```python
from build123d import *

# Parameters (mm, degrees)
SKETCH_1_W               = 90
SKETCH_1_H               = 20
EXTRUDE_1_DEPTH          = 5
SKETCH_4_R               = 13
SKETCH_4_R_2             = 3.75
SKETCH_4_R_3             = 1.8
EXTRUDE_3_DEPTH          = 5
SKETCH_3_R               = 1.8
CUT_EXTRUDE_1_DEPTH      = 48.106262853
SKETCH_4_3_R             = 3.75
SKETCH_4_3_R_2           = 1.8
CUT_EXTRUDE_3_DEPTH      = 48.106262853
EXTRUDE_4_DEPTH          = 10
SKETCH_8_W               = 46.403712297
SKETCH_8_H               = 9.925238464
SKETCH_8_H_2             = 7.991750451
CUT_EXTRUDE_4_DEPTH      = 10
CUT_EXTRUDE_5_DEPTH      = 10
CUT_EXTRUDE_5_DEPTH_BACK = 50.183330509
CUT_EXTRUDE_6_DEPTH      = 10
EXTRUDE_5_DEPTH          = 0.5


with BuildPart() as part:
    # ｽｹｯﾁ1 → ﾎﾞｽ - 押し出し1 (new body)
    with BuildSketch(Plane.XY):
        Rectangle(SKETCH_1_W, SKETCH_1_H)
    extrude(amount=EXTRUDE_1_DEPTH)

    # ｽｹｯﾁ4 → ﾎﾞｽ - 押し出し3 (add)
    with BuildSketch(Plane.XY.offset(5)):
        Circle(SKETCH_4_R)
        Circle(SKETCH_4_R_2, mode=Mode.SUBTRACT)
        with Locations((0, 8.2)):
            Circle(SKETCH_4_R_3, mode=Mode.SUBTRACT)
        with Locations((0, -8.195848947)):
            Circle(SKETCH_4_R_3, mode=Mode.SUBTRACT)
    extrude(amount=-EXTRUDE_3_DEPTH)

    # ｽｹｯﾁ3 → ｶｯﾄ - 押し出し1 (cut, through all)
    with BuildSketch(Plane.XY.offset(5)):
        with Locations((-40, 0)):
            Circle(SKETCH_3_R)
        with Locations((-17, 0)):
            Circle(SKETCH_3_R)
        with Locations((17, 0)):
            Circle(SKETCH_3_R)
        with Locations((40, 0)):
            Circle(SKETCH_3_R)
    extrude(amount=-CUT_EXTRUDE_1_DEPTH, mode=Mode.SUBTRACT)

    # ｽｹｯﾁ4<3> → ｶｯﾄ - 押し出し3 (cut, through all)
    with BuildSketch(Plane.XY.offset(5)):
        Circle(SKETCH_4_3_R)
        with Locations((0, 8.2)):
            Circle(SKETCH_4_3_R_2)
        with Locations((0, -8.195848947)):
            Circle(SKETCH_4_3_R_2)
    extrude(amount=-CUT_EXTRUDE_3_DEPTH, mode=Mode.SUBTRACT)

    # ｽｹｯﾁ6 → ﾎﾞｽ - 押し出し4 (add)
    with BuildSketch(Plane(origin=(0, 0, 0), x_dir=(-1, 0, 0), z_dir=(0, 0, -1))):
        with BuildLine():
            Line((-19.539767143, 10), (-9.797958971, 10))
            ThreePointArc((-9.797958971, 10), (-14, 0), (-9.797958971, -10))
            Line((-9.797958971, -10), (-19.539767143, -10))
            ThreePointArc((-19.539767143, -10), (-21.95, 0), (-19.539767143, 10))
        make_face()
        with BuildLine():
            Line((9.797958971, 10), (19.539767143, 10))
            ThreePointArc((19.539767143, 10), (21.95, 0), (19.539767143, -10))
            Line((19.539767143, -10), (9.797958971, -10))
            ThreePointArc((9.797958971, -10), (14, 0), (9.797958971, 10))
        make_face()
    extrude(amount=EXTRUDE_4_DEPTH)

    # ｽｹｯﾁ8 → ｶｯﾄ - 押し出し4 (cut)
    with BuildSketch(Plane(origin=(0, 0, -10), x_dir=(-1, 0, 0), z_dir=(0, 0, -1))):
        with Locations((0.837844805, 12.962619232)):
            Rectangle(SKETCH_8_W, SKETCH_8_H)
        with Locations((0.837844805, -11.995875226)):
            Rectangle(SKETCH_8_W, SKETCH_8_H_2)
    extrude(amount=-CUT_EXTRUDE_4_DEPTH, mode=Mode.SUBTRACT)

    # ｽｹｯﾁ9 → ｶｯﾄ - 押し出し5 (cut, two sides: drawn at the far end of the back side and taken through both)
    with BuildSketch(Plane.XY.offset(5).offset(-CUT_EXTRUDE_5_DEPTH_BACK)):
        Polygon((8.306623863, -10), (45, -5), (45, -10), align=None)
        Polygon((45, 5), (8.306623863, 10), (45, 10), align=None)
        Polygon((-8.306623863, 10), (-45, 10), (-45, 5), align=None)
        Polygon((-8.306623863, -10), (-45, -10), (-45, -5), align=None)
    extrude(amount=CUT_EXTRUDE_5_DEPTH + CUT_EXTRUDE_5_DEPTH_BACK, mode=Mode.SUBTRACT)

    # ｽｹｯﾁ12 → ｶｯﾄ - 押し出し6 (cut)
    with BuildSketch(Plane(origin=(0, 0, -10), x_dir=(-1, 0, 0), z_dir=(0, 0, -1))):
        with BuildLine():
            Line((-17.5, 3), (17.5, 3))
            ThreePointArc((17.5, 3), (20.5, 0), (17.5, -3))
            Line((17.5, -3), (-17.5, -3))
            ThreePointArc((-17.5, -3), (-20.5, 0), (-17.5, 3))
        make_face()
    extrude(amount=-CUT_EXTRUDE_6_DEPTH, mode=Mode.SUBTRACT)

    # ｽｹｯﾁ13 → ﾎﾞｽ - 押し出し5 (add)
    with BuildSketch(Plane(origin=(0, 0, 0), x_dir=(-1, 0, 0), z_dir=(0, 0, -1))):
        with BuildLine():
            Line((-20.35015639, 8.358895556), (-23.165607924, 7.97524981))
            ThreePointArc((-23.165607924, 7.97524981), (-24.5, 0), (-23.165607924, -7.97524981))
            Line((-23.165607924, -7.97524981), (-20.35015639, -8.358895556))
            ThreePointArc((-20.35015639, -8.358895556), (-22, 0), (-20.35015639, 8.358895556))
        make_face()
        with BuildLine():
            Line((23.165607924, 7.97524981), (20.35015639, 8.358895556))
            ThreePointArc((20.35015639, 8.358895556), (22, 0), (20.35015639, -8.358895556))
            Line((20.35015639, -8.358895556), (23.165607924, -7.97524981))
            ThreePointArc((23.165607924, -7.97524981), (24.5, 0), (23.165607924, 7.97524981))
        make_face()
    extrude(amount=EXTRUDE_5_DEPTH)


solid = part.part
```
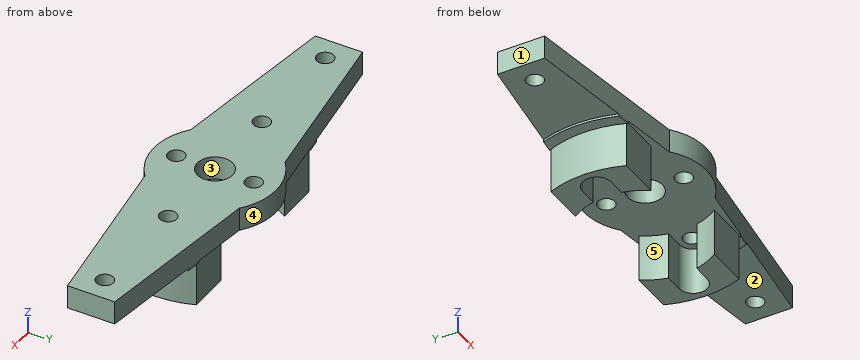
The model under review builds one solid part; all positions refer to its coordinate system, in mm. Face numbers are marked on the shaded views. A direction names the side the tool comes from. Coordinates: 2 decimals unless noted, no trailing zeros. Write each loop counter-clockwise with the first axis right and the second up, starting at its lowest first coordinate (ties: lowest second). Pieces come first, ordered by that corner, then holes.
1) Machinability: for the marked faces 4 and 5, which of the approach directions +Z, -Z, +X, -X, +Y, -Y give a long, thin tool a straight path to every point of the face, cutting with its end or side? Answer none if there is none.
2) To check wall thickness, follow probe 1 along Y at (x, z) = (0, 2.25); probe 2 along X at (y, z) = (-0.5, -4.25); probe 3 along Y at (x, z) = (14.5, -3.5). State the ranges of each line that lie inside material, in increasing order.
3) Clearance check with flat-ended pins moving along their axes: pin 1 Ø2.5 at (x, z) = (16.5, -6.5) entering from +Y; pin 2 Ø13 at (x, y) = (35.5, 3.5) entering from -Z; pin 3 Ø1.1 at (x, z) = (-16, -5) entering from -Y. State where each tip first meets the part, or that it passes through.
4) The part is to be moulded in two halves that separate along X. For the marked faces 1, 2 and 3, say which applies: pulls with the +X half, pulls with the -X half, needs draft (parallel to the pull), parting line crosses it, or undercut.
5) We need section A-A on z = -3.75. State the section outline as (x, y) points, then the cut area to 3 significant figures.
6) We need section D-D on y = 1. Count the separate pieces of the cut face and the enclosed holes in it, then the cut area to 3 significant figures.
7) We need section C-C on z = 1.75. State the section outline as (x, y) points, then the cut area to 3 significant figures.
8) We need section B-B on x = 39.5. State the section outline as (y, z) points.
Answer list:
1. face 4: +Z, -Z, +Y
1. face 5: -Z
2. probe 1: y = -13 to -10, -6.4 to -3.75, 3.75 to 6.4, 10 to 13
2. probe 2: x = -21.94 to -20.46, 20.46 to 21.94
2. probe 3: y = -8 to -3, 3 to 8
3. pin 1: stops at y = 8
3. pin 2: stops at z = 0
3. pin 3: stops at y = -8
4. face 1: pulls with the -X half
4. face 2: needs draft
4. face 3: undercut
5. outline: (-20.44, -8) - (-11.49, -8) arc R14 cw to (-13.67, -3) - (-17.5, -3) arc R3 cw to (-17.5, 3) - (-13.67, 3) arc R14 cw to (-11.49, 8) - (-20.44, 8) arc R21.95 ccw to start; (11.49, -8) - (20.44, -8) arc R21.95 ccw to (20.44, 8) - (11.49, 8) arc R14 cw to (13.67, 3) - (17.5, 3) arc R3 cw to (17.5, -3) - (13.67, -3) arc R14 cw to start
5. area: 193 mm2
6. separate pieces: 6
6. enclosed holes: 0
6. area: 388 mm2
7. outline: (-45, -5) - (-8.31, -10) arc R13 ccw to (8.31, -10) - (45, -5) - (45, 5) - (8.31, 10) arc R13 ccw to (-8.31, 10) - (-45, 5) - close; hole circle Ø3.6 at (-40, 0); hole circle Ø3.6 at (-17, 0); hole circle Ø7.5 at (0, 0); hole circle Ø3.6 at (0, -8.2); hole circle Ø3.6 at (0, 8.2); hole circle Ø3.6 at (17, 0); hole circle Ø3.6 at (40, 0)
7. area: 1,400 mm2
8. outline: (-5.75, 0) - (-1.73, 0) - (-1.73, 5) - (-5.75, 5) - close; (1.73, 0) - (5.75, 0) - (5.75, 5) - (1.73, 5) - close
